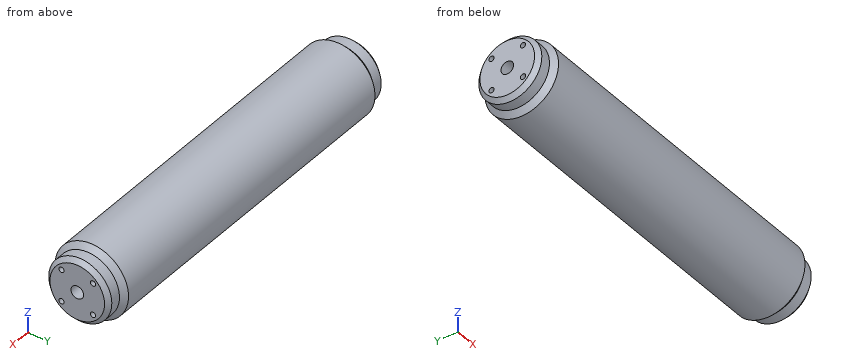
```python
from build123d import *

# Parameters (mm, degrees)
SKETCH1_R                  = 17.5
BOSS_EXTRUDE1_DEPTH        = 80
SKETCH7_R                  = 15
BOSS_EXTRUDE2_DEPTH        = 10
CHAMFER1_SIZE              = 3
CHAMFER2_SIZE              = 2
M3_TAPPED_HOLE1_AT_2_COUNT = 2
M3_TAPPED_HOLE1_AT_2_PITCH = 15
M3_TAPPED_HOLE1_AT_3_COUNT = 2
M3_TAPPED_HOLE1_AT_3_PITCH = 21.213203436
M3_TAPPED_HOLE1_AT_4_COUNT = 2
M3_TAPPED_HOLE1_AT_4_PITCH = 15


with BuildPart() as part:
    # Sketch1 → Boss-Extrude1 (new, symmetric)
    with BuildSketch(Plane(origin=(0, 0, 0), x_dir=(0, 0, -1), z_dir=(1, 0, 0))):
        Circle(SKETCH1_R)
    extrude(amount=BOSS_EXTRUDE1_DEPTH, both=True)

    # Sketch7 → Boss-Extrude2 (add)
    with BuildSketch(Plane.ZY.offset(80)):
        Circle(SKETCH7_R)
    boss_extrude2 = extrude(amount=BOSS_EXTRUDE2_DEPTH)

    # Mirror3: Boss-Extrude2 across plane
    add(boss_extrude2.mirror(Plane(origin=(0, 0, 0), x_dir=(0, 0, 1), z_dir=(1, 0, 0))))

    # Chamfer1
    # the kernel refuses this chamfer: 3 mm, written as the material it adds along each edge
    with BuildSketch(Plane(origin=(80, 0, 0), x_dir=(0, 0, 1), z_dir=(0, -1, 0))) as chamfer1_piece_1_section:
        Polygon((15 + CHAMFER1_SIZE, 0), (15, -CHAMFER1_SIZE), (15, 0), align=None)
    chamfer1_piece_1 = revolve(axis=Axis((80, 0, 0), (-1, 0, 0)), mode=Mode.PRIVATE)
    chamfer1_piece_1 = chamfer1_piece_1 & Plane(origin=(81.737216011, 0, 0), x_dir=(0, 0, -1), z_dir=(1, 0, 0)) * Cylinder(17.5, 72, mode=Mode.PRIVATE)
    add(chamfer1_piece_1)
    with BuildSketch(Plane(origin=(-80, 0, 0), x_dir=(0, 0, 1), z_dir=(0, -1, 0))) as chamfer1_piece_2_section:
        Polygon((15 + CHAMFER1_SIZE, 0), (15, CHAMFER1_SIZE), (15, 0), align=None)
    chamfer1_piece_2 = revolve(axis=Axis((-80, 0, 0), (-1, 0, 0)), mode=Mode.PRIVATE)
    chamfer1_piece_2 = chamfer1_piece_2 & Plane(origin=(-81.737216011, 0, 0), x_dir=(0, 0, -1), z_dir=(1, 0, 0)) * Cylinder(17.5, 72, mode=Mode.PRIVATE)
    add(chamfer1_piece_2)

    # Chamfer2
    chamfer2_edges = [part.edges().sort_by_distance(p)[0] for p in [
        (90, 0, -15),
        (-90, 0, -15),
    ]]
    chamfer(chamfer2_edges, length=CHAMFER2_SIZE)

    # Sketch9 → M3 Tapped Hole1 (revolve, cut)
    with BuildSketch(Plane(origin=(-90, 7.5, -7.5), x_dir=(0, 0, 1), z_dir=(0, 1, 0))):
        Polygon((0, 0), (0, 9.251075774), (1.25, 8.5), (1.25, 0), align=None)
    m3_tapped_hole1 = revolve(axis=Axis((-96.35, 7.5, -7.5), (1, 0, 0)), mode=Mode.SUBTRACT)

    # M3 Tapped Hole1 at 2: M3 Tapped Hole1 ×2
    with Locations(*[(0, 0, i * M3_TAPPED_HOLE1_AT_2_PITCH) for i in range(1, M3_TAPPED_HOLE1_AT_2_COUNT)]):
        add(m3_tapped_hole1, mode=Mode.SUBTRACT)

    # M3 Tapped Hole1 at 3: M3 Tapped Hole1 ×2
    with Locations(*[Vector(0, -0.7071067811865476, 0.7071067811865475) * (i * M3_TAPPED_HOLE1_AT_3_PITCH) for i in range(1, M3_TAPPED_HOLE1_AT_3_COUNT)]):
        add(m3_tapped_hole1, mode=Mode.SUBTRACT)

    # M3 Tapped Hole1 at 4: M3 Tapped Hole1 ×2
    with Locations(*[(0, -i * M3_TAPPED_HOLE1_AT_4_PITCH, 0) for i in range(1, M3_TAPPED_HOLE1_AT_4_COUNT)]):
        add(m3_tapped_hole1, mode=Mode.SUBTRACT)

    # Sketch11 → Ø6.0mm Dowel Hole1 (revolve, cut)
    with BuildSketch(Plane(origin=(-90, 0, 0), x_dir=(0, 0, 1), z_dir=(0, 1, 0))):
        Polygon((0, 0), (0, 10.302581857), (3, 8.5), (3, 0), align=None)
    f_6_0mm_dowel_hole1 = revolve(axis=Axis((-96.35, 0, 0), (1, 0, 0)), mode=Mode.SUBTRACT)

    # Mirror4: M3 Tapped Hole1, Ø6.0mm Dowel Hole1 across plane
    add(m3_tapped_hole1.mirror(Plane(origin=(0, 0, 0), x_dir=(0, 0, 1), z_dir=(1, 0, 0))), mode=Mode.SUBTRACT)
    add(f_6_0mm_dowel_hole1.mirror(Plane(origin=(0, 0, 0), x_dir=(0, 0, 1), z_dir=(1, 0, 0))), mode=Mode.SUBTRACT)

    # Mirror4 copy 1 sketch → Mirror4 copy 1 (revolve, cut)
    with BuildSketch(Plane(origin=(90, 7.5, 7.5), x_dir=(0, 0, 1), z_dir=(0, 1, 0))):
        Polygon((0, 0), (0, -9.251075774), (1.25, -8.5), (1.25, 0), align=None)
    revolve(axis=Axis((96.35, 7.5, 7.5), (1, 0, 0)), mode=Mode.SUBTRACT)

    # Mirror4 copy 2 sketch → Mirror4 copy 2 (revolve, cut)
    with BuildSketch(Plane(origin=(90, -7.5, 7.5), x_dir=(0, 0, 1), z_dir=(0, 1, 0))):
        Polygon((0, 0), (0, -9.251075774), (1.25, -8.5), (1.25, 0), align=None)
    revolve(axis=Axis((96.35, -7.5, 7.5), (1, 0, 0)), mode=Mode.SUBTRACT)

    # Mirror4 copy 3 sketch → Mirror4 copy 3 (revolve, cut)
    with BuildSketch(Plane(origin=(90, -7.5, -7.5), x_dir=(0, 0, 1), z_dir=(0, 1, 0))):
        Polygon((0, 0), (0, -9.251075774), (1.25, -8.5), (1.25, 0), align=None)
    revolve(axis=Axis((96.35, -7.5, -7.5), (1, 0, 0)), mode=Mode.SUBTRACT)


solid = part.part
```
Model file for the job. Use its own axes, mm. Give positions to 0.01 mm unless a question says otherwise; leave off trailing zeros. Order: outer loops, then holes, each group sorted by start corner. A loop starts at its lowest first (then second) coordinate and runs counter-clockwise, first axis right, second up.
1) Pin check, flat tips, straight feed: pin 1 (2 mm diameter, centred on y = 7.5, z = -7.5, fed in from -X); pin 2 (3 mm diameter, centred on x = 30.5, z = 5.5, fed in from -Y); pin 3 (1.5 mm diameter, centred on y = -7.5, z = -7.5, fed in from +X). Stop position of each tip, or through.
2) Saw through at A-A, the plane x = -60.5. Write the cut outline in (y, z), then the cut area to 3 significant figures.
3) Wall check: probe 1 along Y at (x, z) = (88, -7.5); probe 2 along Y at (x, z) = (-85, 0). Give the ranges that are in metal, low to high.
Computed:
1. pin 1: stops at x = -81.35
1. pin 2: stops at y = -17.04
1. pin 3: stops at x = 81.2
2. outline: circle Ø35 at (0, 0)
2. area: 962 mm2
3. probe 1: y = -12.99 to -8.75, -6.25 to 6.25, 8.75 to 12.99
3. probe 2: y = -15 to -3, 3 to 15
